from build123d import *

# Parameters (mm, degrees)
F1_DEPTH = 9.525
F2_R     = 6.6675
F3_DEPTH = 9.526


with BuildPart() as f1:
    # F0 (on Front) → F1 (new body)
    with BuildSketch(Plane.XZ):
        with BuildLine():
            Line((203.2, 0), (171.45, 0))
            ThreePointArc((171.45, 0), (0, 171.45), (-171.45, 0))
            Line((-171.45, 0), (-203.2, 0))
            Line((-203.2, 0), (-203.2, -504.825))
            Line((-203.2, -504.825), (203.2, -504.825))
            Line((203.2, -504.825), (203.2, 0))
        make_face()
    extrude(amount=F1_DEPTH)

    # F2 (on face) → F3 (cut, through all)
    with BuildSketch(Plane.XZ.offset(9.525)):
        with Locations((-180.975, -22.225)):
            Circle(F2_R)
        with Locations((180.975, -22.225)):
            Circle(F2_R)
        with Locations((180.975, -276.225)):
            Circle(F2_R)
        with Locations((-180.975, -276.225)):
            Circle(F2_R)
        with Locations((180.975, -482.6)):
            Circle(F2_R)
        with Locations((-180.975, -482.6)):
            Circle(F2_R)
    extrude(amount=-F3_DEPTH, mode=Mode.SUBTRACT)


solid = f1.part
Geometry check sheet. Reference: the model listing, model coordinates, mm. Round coordinates to 2 decimals unless told otherwise and drop trailing zeros. Loops run counter-clockwise (first coordinate to the right, second up) from the corner with the lowest first, then second, coordinate; pieces in that order, holes last.
Item 1: Cross-section at A-A on z = -482.6. Record the boundary of the cut face in (x, y) (1 decimal).
Item 2: Thickness scan on line 1 (X direction, y = -2.75, z = -482.6); line 2 (Z direction, x = -186, y = -0.5) (3 decimals); line 3 (X direction, y = -0.75, z = 3.5). Record the ranges inside material, lowest first.
Item 3: Cross-section at B-B on y = -6.75. Count the separate pieces of the cut face and the enclosed holes in it, then the cut area to 3 significant figures.
Item 4: Cross-section at C-C on x = -71. Record the boundary of the cut face in (y, z) (3 decimals).
Item 5: Mould release check, pull along X, two halves, no side actions. Record for faces 1 (the cylindrical face through (3.77, -4.7, 171.41)), 2 (the cylindrical face through (187.335, -4.829, -20.222)), 3 (the cylindrical face through (184.559, -4.829, -270.603)), 4 (the flat face through (-3, -9.525, -162)): pulls with the +X half, pulls with the -X half, needs draft (parallel to the pull), parting line crosses it, or undercut.
Item 6: Gauge pin test, flat ends, axial feed: pin 1 (3 mm diameter, centred on x = -159, y = -7.5, fed in from +Z); pin 2 (10.5 mm diameter, centred on x = 180.975, z = -22.225, fed in from -Y); pin 3 (5 mm diameter, centred on x = 184, y = -5, fed in from +Z). Record the tip position at first contact, or that the pin passes through.
Answer sheet:
1. outline: (-203.2, -9.5) - (-187.6, -9.5) - (-187.6, 0) - (-203.2, 0) - close; (-174.3, -9.5) - (174.3, -9.5) - (174.3, 0) - (-174.3, 0) - close; (187.6, -9.5) - (203.2, -9.5) - (203.2, 0) - (187.6, 0) - close
2. line 1: x = -203.2 to -187.64, -174.31 to 174.31, 187.64 to 203.2
2. line 2: z = -504.825 to -486.982, -478.218 to -280.607, -271.843 to -26.607, -17.843 to 0
2. line 3: x = -171.41 to 171.41
3. separate pieces: 1
3. enclosed holes: 6
3. area: 250,000 mm2
4. outline: (-9.525, -504.825) - (0, -504.825) - (0, 156.058) - (-9.525, 156.058) - close
5. face 1: parting line crosses it
5. face 2: undercut
5. face 3: undercut
5. face 4: needs draft
6. pin 1: stops at z = 67.74
6. pin 2: passes through
6. pin 3: stops at z = 0
